Design review of the part built by this model. Coordinates are the model's own, in mm. Coordinates: 2 decimals unless noted, no trailing zeros. Write each loop counter-clockwise with the first axis right and the second up, starting at its lowest first coordinate (ties: lowest second). Pieces come first, ordered by that corner, then holes. Notation, with made-up numbers: (-39, 32.5) - (-27, 32.5) arc R28 cw to (-27, 66.5) - close; hole circle Ø2 at (39, 44.25). An arc over 180 degrees is marked (long way). Answer as CSV lines item,"result". Start each with the question number.
Q1. We need section D-D (y = 28.5). Write out the cut boundary in (x, z) (3 decimals), plus the area to 3 significant figures.
Q2. We need section B-B (y = 16.51). Write out the cut boundary in (x, z) (3 decimals), plus the area to 3 significant figures.
Q3. We need section A-A (z = -88.9). Write out the cut boundary in (x, y), plus the area to 3 significant figures.
Q4. We need section C-C (z = -184.15). Write out the cut boundary in (x, y) (3 decimals).
Q5. For line 1 along Z through (x, y) = (-4.25, 15); line 2 along Z through (x, y) = (-5.5, 17); line 3 along Z through (x, y) = (-1.75, 15), list the stretches that pass through material, from the lowest coordinate up. Write a range as [from, to].
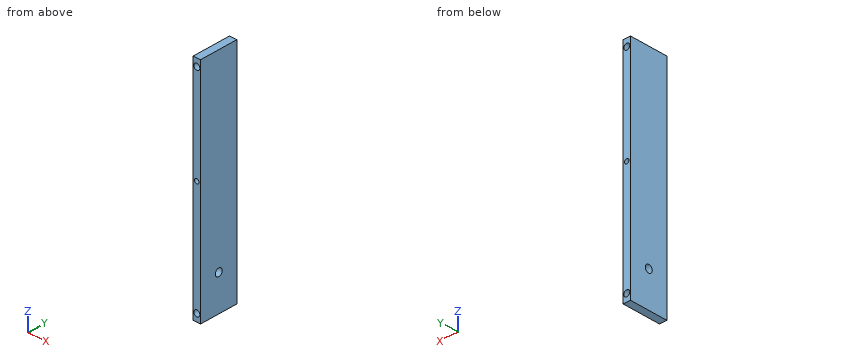
from build123d import *

# Parameters (mm, degrees)
SKETCH1_W           = 6.35
SKETCH1_H           = 33.02
BOSS_EXTRUDE1_DEPTH = 190.5
CUT_EXTRUDE1_REACH  = 195.445
SKETCH2_R           = 3.175
SKETCH3_R           = 2.54
SKETCH3_R_2         = 1.905
CUT_EXTRUDE2_DEPTH  = 194.444805823


with BuildPart() as part:
    # Sketch1 → Boss-Extrude1 (new body)
    with BuildSketch(Plane.XY):
        with Locations((-3.175, 16.51)):
            Rectangle(SKETCH1_W, SKETCH1_H)
    extrude(amount=-BOSS_EXTRUDE1_DEPTH)

    # Sketch2 → Cut-Extrude1 (cut, up to next)
    with BuildSketch(Plane.ZY.offset(6.35), mode=Mode.PRIVATE) as cut_extrude1_sk1:
        with Locations(Location((-160.5000092, 16.51, 0), (0, 0, 270))):
            Circle(SKETCH2_R)
    cut_extrude1_tool1 = extrude(cut_extrude1_sk1.sketch, amount=-CUT_EXTRUDE1_REACH, mode=Mode.PRIVATE) & part.part
    add(cut_extrude1_tool1.solids().sort_by_distance((-6.35, 16.51, -160.500009))[0], mode=Mode.SUBTRACT)

    # Sketch3 → Cut-Extrude2 (cut, through all)
    with BuildSketch(Plane(origin=(0, 33.02, 0), x_dir=(1, 0, 0), z_dir=(0, 1, 0))):
        with Locations(Location((-3.175, 6.35, 0), (0, 0, 270))):
            Circle(SKETCH3_R)
        with Locations(Location((-3.175, 184.15, 0), (0, 0, 270))):
            Circle(SKETCH3_R)
        with Locations(Location((-3.175, 88.9, 0), (0, 0, 270))):
            Circle(SKETCH3_R_2)
    extrude(amount=-CUT_EXTRUDE2_DEPTH, mode=Mode.SUBTRACT)


solid = part.part
Results list:
1,outline,"(-6.35, -190.5) - (0, -190.5) - (0, 0) - (-6.35, 0) - close; hole circle Ø5.08 at (-3.175, -184.15); hole circle Ø5.08 at (-3.175, -6.35); hole circle Ø3.81 at (-3.175, -88.9)"
1,area,"1,160 mm2"
2,outline,"(-6.35, -190.5) - (0, -190.5) - (0, -163.675) - (-6.35, -163.675) - close; (-6.35, -157.325) - (0, -157.325) - (0, 0) - (-6.35, 0) - close; hole circle Ø5.08 at (-3.175, -184.15); hole circle Ø5.08 at (-3.175, -6.35); hole circle Ø3.81 at (-3.175, -88.9)"
2,area,"1,120 mm2"
3,outline,"(-6.35, 0) - (-5.08, 0) - (-5.08, 33.02) - (-6.35, 33.02) - close; (-1.27, 0) - (0, 0) - (0, 33.02) - (-1.27, 33.02) - close"
3,area,"83.9 mm2"
4,outline,"(-6.35, 0) - (-5.715, 0) - (-5.715, 33.02) - (-6.35, 33.02) - close; (-0.635, 0) - (0, 0) - (0, 33.02) - (-0.635, 33.02) - close"
5,line 1,"z = [-190.5, -186.45], [-181.85, -163.29], [-157.71, -90.47], [-87.33, -8.65], [-4.05, 0]"
5,line 2,"z = [-190.5, -185.17], [-183.13, -163.64], [-157.36, -7.37], [-5.33, 0]"
5,line 3,"z = [-190.5, -186.25], [-182.05, -163.29], [-157.71, -90.16], [-87.64, -8.45], [-4.25, 0]"
